Model file for the job. Use its own axes, mm. Face numbers are marked on the shaded views. A direction names the side the tool comes from. Coordinates: 2 decimals unless noted, no trailing zeros. Loops run counter-clockwise (first coordinate to the right, second up) from the corner with the lowest first, then second, coordinate; pieces in that order, holes last. Notation, with made-up numbers: M -40,-36 L -24,-36 A23 cw -24,-8 Z; hole C 62.25,4.5 d2. An arc over 180 degrees is marked long. Write item = value, one per line. Start each with the question number.
Autodesk Inventor part; units mm, degrees
ref_plane "YZ Plane" through (0, 0, 0) normal (1, 0, 0) x (0, 1, 0)
ref_plane "XZ Plane" through (0, 0, 0) normal (0, 1, 0) x (-1, 0, 0)
ref_plane "XY Plane" through (0, 0, 0) normal (0, 0, 1) x (1, 0, 0)
sketch "Sketch1" plane through (0, 0, 0) normal (0, 0, 1) x (1, 0, 0)
  line L0 (0, 0) -> (0, 11.4)
  line L1 (0, 11.4) -> (6, 11.4)
  line L2 (6, 11.4) -> (6, 9.7)
  line L3 (6, 9.7) -> (4, 9.7)
  line L4 (4, 9.7) -> (4, 1.7)
  line L5 (4, 1.7) -> (6, 1.7)
  line L6 (6, 1.7) -> (6, 1)
  line L7 (4, 0) -> (0, 0)
  line L8 (6, 1) -> (4, 0)
  point P0 (6, 0)
  dimension "d0" = 8
  dimension "d1" = 6
  dimension "d2" = 4
  dimension "d3" = 1.7
  dimension "d5" = 1.7
  dimension "d6" = 1
  dimension "d7" = 2
revolve "Revolution1" add sketch "Sketch1" angle 360 about axis through (0, 0, 0) along (0, 1, 0)
sketch "Sketch2" plane through (0, 0, 0) normal (0, -1, 0) x (1, 0, 0)
  line L0 (0, 0) -> (3.4395, 12.8364)
  line L1 (3.4395, 12.8364) -> (-3.4395, 12.8364)
  line L2 (-3.4395, 12.8364) -> (0, 0)
  line L3 (0, 0) -> (0, -2.5884)
  dimension "d8" = 30
extrude "Extrusion1" cut sketch "Sketch2" against normal blind 1.2 draft -60
pattern_circular "Circular Pattern1" count 6 over 360 about axis through (0, -10, 0) along (0, 1, 0) of "Extrusion1"
equation "\"d2\" = d25"
properties part number "Wheel 75 mm - Part 5"
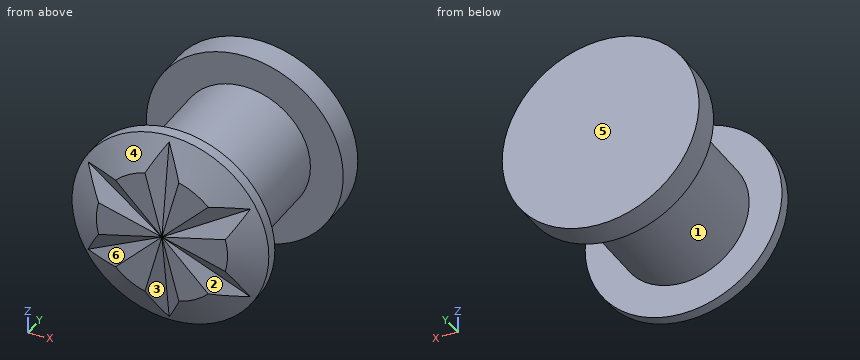
Item 1: Cut at A-A (y = 5). Give the cut face in (x, z), plus the area to 3 significant figures.
Item 2: Cut at B-B (y = 10.25). Give the cut face in (x, z), plus the area to 3 significant figures.
Item 3: 3-axis set-ups, long thin cutter, end or side, ignore diameter. For the marked faces 1, 2 and 3: which of +Z, -Z, +X, -X, +Y, -Y reach the whole face in a straight line?
Item 4: Probe L1, parallel to Y at x = 3.25, z = -3.25; L2, parallel to Y at x = -2, z = -4.75; L3, parallel to Y at x = 0.75, z = -3.25. List the from-to ranges inside material, lowest first.
Item 5: Pin check, flat tips, straight feed: pin 1 Ø3 at (x, z) = (4.5, 4) entering from -Y; pin 2 Ø5 at (y, z) = (5.5, 1) entering from -X; pin 3 Ø5 at (y, z) = (10, 3) entering from +X. Stop position of each tip, or through.
Item 6: Pull direction Z, two halves, no side cores. Call the marked faces 4, 5 and 6: +Z half, -Z half, draft (parallel to the pull), parting line (faces both ways), or undercut.
Reported:
q1.outline = C 0,0 d8
q1.area = 50.3 mm^2
q2.outline = C 0,0 d12
q2.area = 113 mm^2
q3.face_1 = none
q3.face_2 = -Y
q3.face_3 = -Z, -Y
q4.L1 = 0.3 to 1.7, 9.7 to 11.4
q4.L2 = 0.58 to 1.7, 9.7 to 11.4
q4.L3 = 0.07 to 11.4
q5.pin_1 = 0.26
q5.pin_2 = -4
q5.pin_3 = 5.98
q6.face_4 = parting line
q6.face_5 = draft
q6.face_6 = undercut
